Could you check a few things on this drawing? It's one solid part, dimensions in mm from its lowest x, y, z. A direction names the side the tool comes from. Coordinates: 2 decimals unless noted, no trailing zeros. Write each loop counter-clockwise with the first axis right and the second up, starting at its lowest first coordinate (ties: lowest second). Pieces come first, ordered by that corner, then holes.
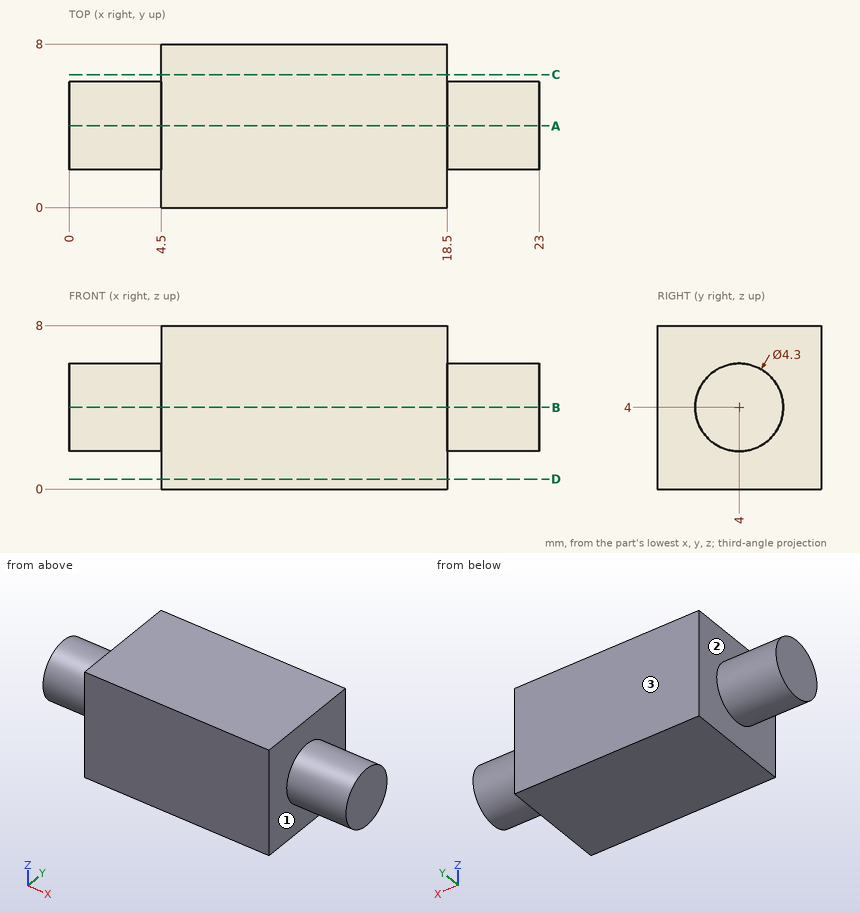
1) I need wall thicknesses on probe 1 along X at (y, z) = (4.5, 6.5); probe 2 along Z at (x, y) = (3.5, 5.5); probe 3 along Y at (x, z) = (20.75, 3.25). Which ranges of each line are inside material? Lowest first, please.
Values follow:
probe 1: x = 4.5 to 18.5
probe 2: z = 2.46 to 5.54
probe 3: y = 1.99 to 6.01
2) On a 3-axis mill with a long thin cutter (end or side, diameter ignored), from which of +Z, -Z, +X, -X, +Y, -Y can I reach the whole of each face in a straight line? I mean the marked faces 1, 2 and 3. Say none if no direction works.
Values follow:
face 1: +X
face 2: -X
face 3: +Z, -Z, +X, -X, +Y
3) Will this pin go through, and if not, where does the flat tip stop? pin 1 (4 mm diameter, centred on y = 2, z = 2.5, fed in from -X).
Values follow:
pin 1: stops at x = 0
4) Imagine slicing it at A-A on y = 4. Please give me the cut outline in (x, z).
Values follow:
outline: (0, 1.85) - (4.5, 1.85) - (4.5, 0) - (18.5, 0) - (18.5, 1.85) - (23, 1.85) - (23, 6.15) - (18.5, 6.15) - (18.5, 8) - (4.5, 8) - (4.5, 6.15) - (0, 6.15) - close
5) Imagine slicing it at C-C on y = 6.5. Please give me the cut outline in (x, z).
Values follow:
outline: (4.5, 0) - (18.5, 0) - (18.5, 8) - (4.5, 8) - close
